```python
from build123d import *

# Parameters (mm, degrees)
SKETCH1_W           = 76.2
SKETCH1_H           = 76.2
SKETCH1_R           = 31.75
BOSS_EXTRUDE1_DEPTH = 3.175
CUT_EXTRUDE1_REACH  = 55.975
SKETCH2_R           = 2.665
CIRPATTERN1_COUNT   = 4
FILLET1_R           = 6.35


with BuildPart() as part:
    # Sketch1 → Boss-Extrude1 (new body)
    with BuildSketch(Plane(origin=(0, 0, 0), x_dir=(1, 0, 0), z_dir=(0, 1, 0))):
        Rectangle(SKETCH1_W, SKETCH1_H)
        with Locations(Location((0, 0, 0), (0, 0, 270))):
            Circle(SKETCH1_R, mode=Mode.SUBTRACT)
    extrude(amount=BOSS_EXTRUDE1_DEPTH)

    # Sketch2 → Cut-Extrude1 (cut, up to next)
    with BuildSketch(Plane(origin=(0, 3.175, 0), x_dir=(1, 0, 0), z_dir=(0, 1, 0)), mode=Mode.PRIVATE) as cut_extrude1_sk1:
        with Locations(Location((31.430896424, 31.430896424, 0), (0, 0, 270))):
            Circle(SKETCH2_R)
    cut_extrude1_tool1 = extrude(cut_extrude1_sk1.sketch, amount=-CUT_EXTRUDE1_REACH, mode=Mode.PRIVATE) & part.part
    cut_extrude1 = cut_extrude1_tool1.solids().sort_by_distance((31.430896, 3.175, -31.430896))[0]
    add(cut_extrude1, mode=Mode.SUBTRACT)

    # CirPattern1: Cut-Extrude1 ×4 about axis
    cirpattern1_axis = Axis((0, 0, 0), (0, 1, 0))
    for i in range(1, CIRPATTERN1_COUNT):
        add(cut_extrude1.rotate(cirpattern1_axis, i * 360 / CIRPATTERN1_COUNT), mode=Mode.SUBTRACT)

    # Fillet1
    fillet1_edges = [part.edges().sort_by_distance(p)[0] for p in [
        (38.1, 1.5875, 38.1),
        (-38.1, 1.5875, 38.1),
        (-38.1, 1.5875, -38.1),
        (38.1, 1.5875, -38.1),
    ]]
    fillet(fillet1_edges, radius=FILLET1_R)


solid = part.part
```
Work out the finished part from the listing and answer in its coordinate system (mm). Coordinates: 2 decimals unless noted, no trailing zeros. Order: outer loops, then holes, each group sorted by start corner. A loop starts at its lowest first (then second) coordinate and runs counter-clockwise, first axis right, second up. Notation, with made-up numbers: (-7.5, 85.5) - (45.5, 85.5) arc R19 ccw to (45.5, 94.5) - close; hole circle Ø2 at (-3.5, -25). An arc over 180 degrees is marked (long way). Answer as a JSON object with one key per item and string values.
1. Consider line 1 (X direction, y = 1.5, z = 0); line 2 (Z direction, x = -32.5, y = 2.45); line 3 (X direction, y = 1.05, z = -17). Determine where each line is inside the solid, lowest interval first.
Output values:
{"line 1": "x = -38.1 to -31.75, 31.75 to 38.1", "line 2": "z = -38.06 to -33.87, -28.99 to 28.99, 33.87 to 38.06", "line 3": "x = -38.1 to -26.82, 26.82 to 38.1"}
2. This flat-tipped pin is pushed along its axis until it touches: P1, Ø5, axis at x = 31.43, z = -31.43, coming from the +Y side (1 decimal). Where does it stop, or does it pass through?
Output values:
{"P1": "passes through"}
3. Find section D-D on y = 0.75. Determine the outline of the cut face in (x, z) (3 decimals), plus the area to 3 significant figures.
Output values:
{"outline": "(-38.1, -31.75) arc R6.35 ccw to (-31.75, -38.1) - (31.75, -38.1) arc R6.35 ccw to (38.1, -31.75) - (38.1, 31.75) arc R6.35 ccw to (31.75, 38.1) - (-31.75, 38.1) arc R6.35 ccw to (-38.1, 31.75) - close; hole circle Ø5.33 at (-31.431, -31.431); hole circle Ø5.33 at (-31.431, 31.431); hole circle Ø63.5 at (0, 0); hole circle Ø5.33 at (31.431, -31.431); hole circle Ø5.33 at (31.431, 31.431)", "area": "2,520 mm²"}
4. Find section C-C on z = -30.5. Determine the outline of the cut face in (x, y) (3 decimals).
Output values:
{"outline": "(-38.1, 0) - (-33.928, 0) - (-33.928, 3.175) - (-38.1, 3.175) - close; (-28.934, 0) - (-8.821, 0) - (-8.821, 3.175) - (-28.934, 3.175) - close; (8.821, 0) - (28.934, 0) - (28.934, 3.175) - (8.821, 3.175) - close; (33.928, 0) - (38.1, 0) - (38.1, 3.175) - (33.928, 3.175) - close"}
5. The mould has two halves that part along Z. Classify faces 1 (the face through (-32.01, 1.61, -28.83)), 2 (the face through (-34, 3.175, -1)), 3 (the face through (36.19, 1.61, -36.29)): +Z half, -Z half, draft (parallel to the pull), parting line (faces both ways), or undercut.
Output values:
{"face 1": "undercut", "face 2": "draft", "face 3": "-Z half"}
6. Find section B-B on x = 8.5. Determine the outline of the cut face in (y, z) (3 decimals).
Output values:
{"outline": "(0, -38.1) - (3.175, -38.1) - (3.175, -30.591) - (0, -30.591) - close; (0, 30.591) - (3.175, 30.591) - (3.175, 38.1) - (0, 38.1) - close"}
7. Find section A-A on z = 0. Determine the outline of the cut face in (x, y) (3 decimals), plus the area to 3 significant figures.
Output values:
{"outline": "(-38.1, 0) - (-31.75, 0) - (-31.75, 3.175) - (-38.1, 3.175) - close; (31.75, 0) - (38.1, 0) - (38.1, 3.175) - (31.75, 3.175) - close", "area": "40.3 mm²"}
